Part model, mm, in its own coordinate system. A direction names the side the tool comes from. Give positions to 0.01 mm unless a question says otherwise; leave off trailing zeros. Loops run counter-clockwise (first coordinate to the right, second up) from the corner with the lowest first, then second, coordinate; pieces in that order, holes last. Notation, with made-up numbers: (9.5, 66) -> (47.5, 66) arc R9 cw to (47.5, 74) -> close; hole circle Ø6 at (15, 65.5). An arc over 180 degrees is marked (long way). Write item = value, one per line.
from build123d import *

# Parameters (mm, degrees)
F1_DEPTH = 120.65
F2_R     = 1.98374
F3_R     = 3.69316
F4_R     = 3.96875
F5_R     = 0.762
F6_R     = 1.8288
F7_DEPTH = 1.70942


with BuildPart() as f1:
    # F0 (on Top) → F1 (new body)
    with BuildSketch(Plane.XY):
        Polygon((0, -13.29058), (0, 0), (9.92124, 0), (9.92124, 1.70942), (-1.70942, 1.70942), (-1.70942, -11.58116), (-16.70942, -11.58116), (-16.70942, -13.29058), align=None)
    extrude(amount=F1_DEPTH)

    # F2
    f2_edges = [f1.edges().sort_by_distance(p)[0] for p in [
        (0, 0, 60.325),
        (-1.70942, -11.58116, 60.325),
    ]]
    fillet(f2_edges, radius=F2_R)

    # F3
    f3_edges = [f1.edges().sort_by_distance(p)[0] for p in [
        (0, -13.29058, 60.325),
        (-1.70942, 1.70942, 60.325),
    ]]
    fillet(f3_edges, radius=F3_R)

    # F4
    f4_edges = [f1.edges().sort_by_distance(p)[0] for p in [
        (9.92124, 0.85471, 120.65),
        (9.92124, 0.85471, 0),
    ]]
    fillet(f4_edges, radius=F4_R)

    # F5
    f5_edges = [f1.edges().sort_by_distance(p)[0] for p in [
        (-16.70942, -12.43587, 0),
        (-16.70942, -12.43587, 120.65),
    ]]
    fillet(f5_edges, radius=F5_R)

    # F6 (on face) → F7 (cut, through all)
    with BuildSketch(Plane.XZ):
        with Locations((5.95249, 116.68125)):
            Circle(F6_R)
        with Locations((5.95249, 3.96875)):
            Circle(F6_R)
        with Locations((5.95249, 60.325)):
            Circle(F6_R)
    extrude(amount=-F7_DEPTH, mode=Mode.SUBTRACT)


solid = f1.part
1) Slice it at C-C, the plane y = -7. List the corners of the cut face in (x, z), and give its area (3 significant figures).
Resolved:
outline = (-1.71, 0) -> (0, 0) -> (0, 120.65) -> (-1.71, 120.65) -> close
area = 206 mm²
2) Which spindle directions (+Z, -Z, +X, -X, +Y, -Y) get a long thin tool onto all of the face, cutting with end or side? Do faces 5 (the face through (-1.709, -6, 59)), 6 (the face through (-10, -13.291, 59)), 7 (the face through (4, 0, 59)). Say none if no direction does.
Resolved:
face_5 = +Z, -Z, -X, +Y
face_6 = +Z, -Z, +X, -X, -Y
face_7 = +Z, -Z, +X, -Y
3) Drop flat-ended pins along their axis: P1, Ø6, axis at x = 5.95, z = 3.97, coming from the -Y side; P2, Ø4, axis at y = -7, z = 103.5, coming from the +X side; P3, Ø5, axis at x = -5.5, z = 84, coming from the +Y side. Give the stop position or say it passes through.
Resolved:
P1 = 0
P2 = 0
P3 = -11.46
4) Slice it at B-B, the plane x = -12. List the corners of the cut face in (y, z).
Resolved:
outline = (-13.29, 0) -> (-11.58, 0) -> (-11.58, 120.65) -> (-13.29, 120.65) -> close
5) Pull direction X, two halves, no side cores. Call faces 1 (the face through (5.556, 0.843, 114.896)), 2 (the face through (8.728, 0.867, 119.518)), 3 (the face through (5.71, 0.84, 5.78)), 4 (the face through (-1, -7, 120.65)): pulls with the +X half, pulls with the -X half, needs draft (parallel to the pull), parting line crosses it, or undercut.
Resolved:
face_1 = undercut
face_2 = pulls with the +X half
face_3 = undercut
face_4 = needs draft
6) Slice it at A-A, the plane z = 50. List the corners of the cut face in (x, y).
Resolved:
outline = (-16.71, -13.29) -> (-3.69, -13.29) arc R3.69 ccw to (0, -9.6) -> (0, -1.98) arc R1.98 cw to (1.98, 0) -> (9.92, 0) -> (9.92, 1.71) -> (1.98, 1.71) arc R3.69 ccw to (-1.71, -1.98) -> (-1.71, -9.6) arc R1.98 cw to (-3.69, -11.58) -> (-16.71, -11.58) -> close
7) Drill centre lines: line 1 along Y through (x, z) = (-7.5, 61); line 2 along Y through (x, z) = (7.5, 7.5); line 3 along X through (y, z) = (-7.25, 104). Where is each one in solid material? Low to high. Write a range as [from, to].
Resolved:
line_1 = [-13.29, -11.58]
line_2 = [0, 1.71]
line_3 = [-1.71, 0]
